Study the drawing (mm; zero at the part's minimum x, y, z) and answer. A direction names the side the tool comes from. Round coordinates to 2 decimals unless told otherwise and drop trailing zeros. Order: outer loops, then holes, each group sorted by start corner. A loop starts at its lowest first (then second) coordinate and runs counter-clockwise, first axis right, second up. Notation, with made-up numbers: M 22.25,80 L 69.25,80 A19 cw 69.25,91 Z; hole C -36,-32 d3. An arc over 180 degrees is marked long. Put each result on its own line as item: value. Start each with the question number.
1. Each of these flat-tipped pins is pushed along its axis until it touches: pin 1 Ø1 at (x, z) = (91.5, 65.5) entering from +Y; pin 2 Ø3 at (x, z) = (53, 43) entering from -Y; pin 3 Ø2 at (x, z) = (87, 88.5) entering from +Y. Where does it stop, or does it pass through?
2. The part is cut by section C-C (y = 83.5). Give the vertices of the cut face in (x, z).
3. The mould has two halves that part along X. Classify the marked faces 1, 2 and 3: +X half, -X half, draft (parallel to the pull), parting line (faces both ways), or undercut.
4. The part is cut by section B-B (x = 97). Give the vertices of the cut face in (y, z) (1 decimal), then the cut area to 3 significant figures.
5. Consider line 1 (Y direction, x = 65.5, z = 77) (1 decimal); line 2 (X direction, y = 29, z = 30) (1 decimal); line 3 (X direction, y = 98.5, z = 92.5) (1 decimal). Determine where each line is inside the solid, lowest interval first.
6. Which of the six approach directions +Z, -Z, +X, -X, +Y, -Y give full straight-line access (tool end or side, diameter ignored) to the marked faces 4 and 5?
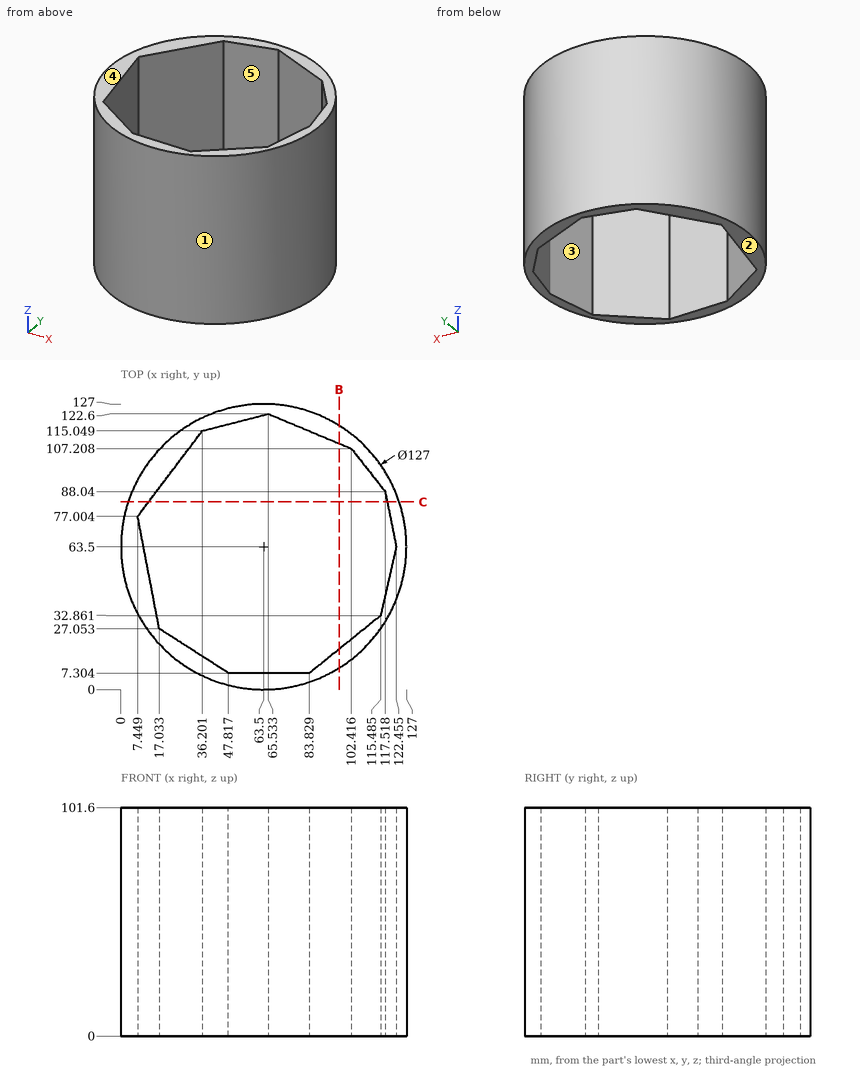
Resolved:
1. pin 1: y = 120.74
1. pin 2: y = 0.64
1. pin 3: y = 122.88
2. outline: M 3.23,0 L 12.36,0 L 12.36,101.6 L 3.23,101.6 Z; M 118.43,0 L 123.77,0 L 123.77,101.6 L 118.43,101.6 Z
3. face 1: parting line
3. face 2: draft
3. face 3: undercut
4. outline: M 9.6,0 L 17.9,0 L 17.9,101.6 L 9.6,101.6 Z; M 109.5,0 L 117.4,0 L 117.4,101.6 L 109.5,101.6 Z
4. area: 1,660 mm2
5. line 1: 0 to 7.3, 122.6 to 127
5. line 2: 10.2 to 16.7, 110.7 to 116.8
5. line 3: 10.5 to 23.7, 109.3 to 116.5
6. face 4: +Z, +X, -X, +Y, -Y
6. face 5: +Z, -Z
